from build123d import *

# Parameters (mm, degrees)
F1_DEPTH = 10


with BuildPart() as f1:
    # F0 (on Front) → F1 (new body)
    with BuildSketch(Plane.XZ):
        with BuildLine():
            ThreePointArc((-37.644739, -19.448335), (-33.644739, -15.448335), (-29.644739, -19.448335))
            Line((-29.644739, -19.448335), (-24.644739, -19.448335))
            Line((-24.644739, -19.448335), (-24.644739, -9.448335))
            Line((-24.644739, -9.448335), (7.460523, -9.448335))
            Line((7.460523, -9.448335), (7.460523, -19.448335))
            Line((7.460523, -19.448335), (32.355261, -19.448335))
            ThreePointArc((32.355261, -19.448335), (36.355261, -15.448335), (40.355261, -19.448335))
            Line((40.355261, -19.448335), (46.355261, -19.448335))
            Line((46.355261, -19.448335), (46.355261, 0.551665))
            Line((46.355261, 0.551665), (-43.644739, 0.551665))
            Line((-43.644739, 0.551665), (-43.644739, -19.448335))
            Line((-43.644739, -19.448335), (-37.644739, -19.448335))
        make_face()
    extrude(amount=F1_DEPTH)


solid = f1.part
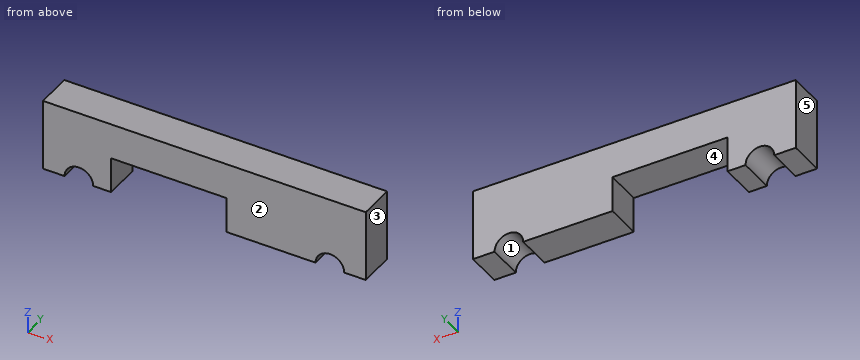
For this review, take the finished solid that the model builds, in its own axes (mm). Face numbers are marked on the shaded views. A direction names the side the tool comes from. Round coordinates to 2 decimals unless told otherwise and drop trailing zeros. Write each loop counter-clockwise with the first axis right and the second up, starting at its lowest first coordinate (ties: lowest second). Pieces come first, ordered by that corner, then holes. Notation, with made-up numbers: M 73,27 L 92,27 A32 ccw 92,56 Z; hole C -31,77 d4. An arc over 180 degrees is marked long. Write item = value, one per line. Start each with the question number.
(1) For the marked faces 4 and 5, list the 3-axis set-ups (+Z, -Z, +X, -X, +Y, -Y) from which the entire face can be reached by the end or side of a thin tool; tool diameter is ignored.
(2) For line 1 along X through (y, z) = (-1, -11.5); line 2 along X through (y, z) = (-2, -15.75); line 3 along X through (y, z) = (-0.5, -16.5), list the stretches that pass through material, from the lowest coordinate up.
(3) The part is to be moulded in two halves that separate along X. For the marked faces 1, 2 and 3, say which applies: +X half, -X half, draft (parallel to the pull), parting line (faces both ways), or undercut.
(4) We need section C-C (x = -6.5). Give the boundary of the cut face in (y, z), then the cut area to 3 significant figures.
(5) We need section B-B (y = -3.25). Give the boundary of the cut face in (x, z), then the cut area to 3 significant figures.
(6) Clearance check with flat-ended pins moving along their axes: pin 1 Ø2 at (x, z) = (13, -12) entering from +Y; pin 2 Ø1 at (x, z) = (37, -17) entering from -Y. State where each tip first meets the part, or that it passes through.
(7) We need section A-A (z = -14.25). Give the boundary of the cut face in (x, y), then the cut area to 3 significant figures.
Results found:
q1.face_4 = -Z, +Y, -Y
q1.face_5 = +Z, -Z, -X, +Y, -Y
q2.line_1 = -43.64 to -24.64, 7.46 to 46.36
q2.line_2 = -43.64 to -35.17, -32.12 to -24.64, 7.46 to 34.83, 37.88 to 46.36
q2.line_3 = -43.64 to -36.35, -30.94 to -24.64, 7.46 to 33.65, 39.06 to 46.36
q3.face_1 = undercut
q3.face_2 = draft
q3.face_3 = +X half
q4.outline = M -10,-9.45 L 0,-9.45 L 0,0.55 L -10,0.55 Z
q4.area = 100 mm²
q5.outline = M -43.64,-19.45 L -37.64,-19.45 A4 cw -29.64,-19.45 L -24.64,-19.45 L -24.64,-9.45 L 7.46,-9.45 L 7.46,-19.45 L 32.36,-19.45 A4 cw 40.36,-19.45 L 46.36,-19.45 L 46.36,0.55 L -43.64,0.55 Z
q5.area = 1,430 mm²
q6.pin_1 = 0
q6.pin_2 = through
q7.outline = M -43.64,-10 L -24.64,-10 L -24.64,0 L -43.64,0 Z; M 7.46,-10 L 46.36,-10 L 46.36,0 L 7.46,0 Z
q7.area = 579 mm²
